The listing builds one solid part. Answer for the finished solid, in the listing's coordinates (mm). A direction names the side the tool comes from. Give positions to 0.01 mm unless a question says otherwise; leave off trailing zeros. Loops run counter-clockwise (first coordinate to the right, second up) from the corner with the lowest first, then second, coordinate; pieces in that order, holes last. Notation, with made-up numbers: M 42.25,89.25 L 48.25,89.25 A20 ccw 48.25,94.25 Z; hole C 23,-28.75 d4. An arc over 180 degrees is marked long. One line per item, written item: value. Start each with the question number.
Q1. Flat-ended cylindrical pins translate along their axes: pin 1 (11 mm diameter, centred on x = -13, z = -12.5, fed in from +Y); pin 2 (5 mm diameter, centred on x = -7.5, y = 5, fed in from -Z); pin 3 (10 mm diameter, centred on y = -7.5, z = 2, fed in from +X). Find the tip coordinate at first contact, or state that the pin passes through.
Q2. A cutting plane is placed at A-A, the plane y = 0.75. Determine the outline of the cut face in (x, z), and give its area (3 significant figures).
Q3. For faces 5 (the cylindrical face through (-0.291, -13.247, -2.605)), 6 (the flat face through (3.25, 2, 2)), 7 (the flat face through (-9.25, 5, 2)), 8 (the cylindrical face through (0.14, -6.25, -23.21)), determine the directions among +Z, -Z, +X, -X, +Y, -Y from which every point of the face is accessible in a straight line to the end or side of a thin tool.
Q4. A cutting plane is placed at B-B, the plane z = -14. Determine the outline of the cut face in (x, y), and give its area (3 significant figures).
Q5. Consider L1, parallel to X at y = 6, z = 0.5; L2, parallel to Z at x = -6.5, y = -0.25; L3, parallel to Z at x = -9, y = -14. Determine where each line is inside the solid, lowest interval first.
Q6. The mould has two halves that part along Z. Classify faces 1 (the flat face through (6, 4, 0)), 2 (the cylindrical face through (-0.203, -9.248, -17.965)), 3 (the flat face through (9.25, 5, 2)), 4 (the flat face through (0, -14, -10)): +Z half, -Z half, draft (parallel to the pull), parting line (faces both ways), or undercut.
Q7. A cutting plane is placed at D-D, the plane y = -7. Determine the outline of the cut face in (x, z).
Q8. A cutting plane is placed at C-C, the plane x = 0. Determine the outline of the cut face in (y, z).
from build123d import *

# Parameters (mm, degrees)
EXTRUDE_1_DEPTH = 5
EXTRUDE_3_DEPTH = 10
EXTRUDE_4_DEPTH = 10.5
EXTRUDE_6_DEPTH = 15
EXTRUDE_7_DEPTH = 5.5
EXTRUDE_8_DEPTH = 5.5


with BuildPart() as part:
    # Sketch 1 → Extrude 1 (new body)
    with BuildSketch(Plane.XY):
        with BuildLine():
            Line((-3.25, 9.25), (-9.25, 9.25))
            Line((-9.25, 9.25), (-9.25, -1.7e-08))
            ThreePointArc((-9.25, -1.7e-08), (9e-09, -9.25), (9.25, 0))
            Line((9.25, 0), (9.25, 9.25))
            Line((9.25, 9.25), (3.25, 9.25))
            Line((3.25, 9.25), (3.25, -5.338539126))
            ThreePointArc((3.25, -5.338539126), (0, -6.25), (-3.25, -5.338539126))
            Line((-3.25, -5.338539126), (-3.25, 9.25))
        make_face()
    extrude(amount=EXTRUDE_1_DEPTH)

    # Sketch 1_4 → Extrude 3 (add)
    with BuildSketch(Plane.XY):
        with BuildLine():
            Line((-6.25, 0), (-9.25, 0))
            ThreePointArc((-9.25, -1.7e-08), (9e-09, -9.25), (9.25, 0))
            Line((9.25, 0), (6.25, 0))
            ThreePointArc((6.25, 0), (9e-09, -6.25), (-6.25, -1.8e-08))
        make_face()
    extrude(amount=-EXTRUDE_3_DEPTH)



with BuildPart() as body_2:
    # Sketch 2 → Extrude 4 (new body)
    with BuildSketch(Plane(origin=(0, 0, -10), x_dir=(-1, 0, 0), z_dir=(0, 0, -1))):
        with BuildLine():
            ThreePointArc((9.25, 0), (0, -9.25), (-9.25, 0))
            Line((-9.25, 0), (-16.35, 0))
            Line((-16.35, 0), (-16.35, -15))
            Line((-16.35, -15), (16.35, -15))
            Line((16.35, -15), (16.35, 0))
            Line((16.35, 0), (9.25, 0))
        make_face()
    extrude(amount=EXTRUDE_4_DEPTH)


with BuildPart() as part_1:
    add(part.part)

    add(body_2.part)  # Extrude 6 merges body 2
    # Sketch 5 → Extrude 6 (add)
    with BuildSketch(Plane.XY.offset(-10)):
        with BuildLine():
            ThreePointArc((9.25, 0), (0, -9.25), (-9.25, 0))
            Line((-9.25, 0), (-13.25, 0))
            ThreePointArc((-13.25, 0), (0, -13.25), (13.25, 0))
            Line((13.25, 0), (9.25, 0))
        make_face()
    extrude(amount=EXTRUDE_6_DEPTH)

    # Sketch 6 → Extrude 7 (add)
    with BuildSketch(Plane(origin=(0, 0, -10), x_dir=(-1, 0, 0), z_dir=(0, 0, -1))):
        with BuildLine():
            Line((9.25, 0), (6.25, 0))
            ThreePointArc((6.25, 0), (0, -6.25), (-6.25, 0))
            Line((-6.25, 0), (-9.25, 0))
            ThreePointArc((-9.25, 0), (0, -9.25), (9.25, 0))
        make_face()
    extrude(amount=EXTRUDE_7_DEPTH)

    # Sketch 7 → Extrude 8 (add)
    with BuildSketch(Plane(origin=(0, 0, -20.5), x_dir=(-1, 0, 0), z_dir=(0, 0, -1))):
        with BuildLine():
            Line((16.35, 0), (16.35, -15))
            Line((16.35, -15), (-16.35, -15))
            Line((-16.35, -15), (-16.35, 0))
            Line((-16.35, 0), (-6.25, 0))
            ThreePointArc((-6.25, 0), (0, -6.25), (6.25, 0))
            Line((6.25, 0), (16.35, 0))
        make_face()
    extrude(amount=EXTRUDE_8_DEPTH)


solid = part_1.part
Answer block:
1. pin 1: y = 0
1. pin 2: z = 0
1. pin 3: x = 13.01
2. outline: M -9.25,0 L -3.25,0 L -3.25,5 L -9.25,5 Z; M 3.25,0 L 9.25,0 L 9.25,5 L 3.25,5 Z
2. area: 60.0 mm^2
3. face 5: +Z, -Y
3. face 6: +Z, -Z, +Y
3. face 7: +Z, -Z, -X, +Y
3. face 8: -Z, +Y
4. outline: M -16.35,-15 L 16.35,-15 L 16.35,0 L 6.25,0 A6.25 cw -6.25,0 L -16.35,0 Z
4. area: 429 mm^2
5. L1: -9.25 to -3.25, 3.25 to 9.25
5. L2: -26 to -20.5, -15.5 to 5
5. L3: -26 to -10
6. face 1: -Z half
6. face 2: undercut
6. face 3: draft
6. face 4: +Z half
7. outline: M -16.35,-26 L 16.35,-26 L 16.35,-10 L 11.25,-10 L 11.25,5 L -11.25,5 L -11.25,-10 L -16.35,-10 Z; hole M -6.05,-20.5 L 6.05,-20.5 L 6.05,-15.5 L -6.05,-15.5 Z
8. outline: M -15,-26 L -6.25,-26 L -6.25,-20.5 L -9.25,-20.5 L -9.25,-15.5 L -6.25,-15.5 L -6.25,5 L -13.25,5 L -13.25,-10 L -15,-10 Z
